For this review, take the finished solid that the model builds, in its own axes (mm). Face numbers are marked on the shaded views. A direction names the side the tool comes from. Give positions to 0.01 mm unless a question says otherwise; leave off trailing zeros. Loops run counter-clockwise (first coordinate to the right, second up) from the corner with the lowest first, then second, coordinate; pieces in that order, holes last. Notation, with made-up numbers: (60, -39.75) - (84, -39.75) arc R11 ccw to (84, -24.75) - close; hole circle Ø4 at (-25, 64). An arc over 180 degrees is marked (long way). Put each result on its own line as item: value. Start each with the question number.
Autodesk Inventor part; units mm, degrees
ref_plane "YZ Plane" through (0, 0, 0) normal (1, 0, 0) x (0, 1, 0)
ref_plane "XZ Plane" through (0, 0, 0) normal (0, 1, 0) x (-1, 0, 0)
ref_plane "XY Plane" through (0, 0, 0) normal (0, 0, 1) x (1, 0, 0)
sketch "Sketch1" plane through (0, 0, 0) normal (0, 1, 0) x (-1, 0, 0)
  line L0 (4, 2.5) -> (-4, 2.5)
  line L1 (-4, 2.5) -> (-4, -2.5)
  line L2 (-4, -2.5) -> (4, -2.5)
  line L3 (4, -2.5) -> (4, 2.5)
  line L4 (4, 2.5) -> (-4, -2.5) construction
  line L5 (-4, 2.5) -> (4, -2.5) construction
  circle A0 centre (2, 0) radius 0.889
  circle A1 centre (-1, 0) radius 0.889
  line L6 (2, -0.889) -> (-1, -0.889)
  line L7 (2, 0.889) -> (-1, 0.889)
  point P0 (0, 0)
  point P1 (0, 0)
  point P2 (0, 0)
  point P3 (0, 0)
  dimension "d19" = 8
  dimension "d20" = 5
  dimension "d21" = 1.778
  dimension "d22" = 2
  dimension "d23" = 3
extrude "Extrusion1" add sketch "Sketch1" along normal mid plane 2
sketch "Sketch4" plane through (-4, 1, 2.5) normal (0, 0, 1) x (1, 0, 0)
  line L0 (8, -2) -> (6.5, -2)
  line L1 (6.5, -2) -> (6.5, -1.5)
  line L2 (6.5, -1.5) -> (8, -1.5)
  line L3 (8, -1.5) -> (8, -2)
  line L4 (8, -2) -> (0, -2)
  line L5 (8, -2) -> (8, 0)
  point P0 (4, -1)
  dimension "d24" = 0.5
  dimension "d25" = 1.5
extrude "Extrusion3" cut sketch "Sketch4" against normal through all
fillet "Fillet2" radius 0.5 4 edges at (-4, 0, 2.5) (-4, 0, -2.5) (4, 0.25, 2.5) (4, 0.25, -2.5)
properties part number "ChipClip"
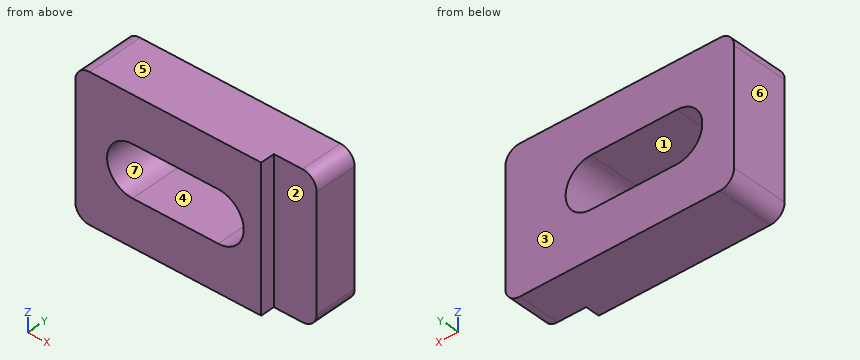
1) Mouldability with a two-part tool opening along Z and no side actions: class the marked faces 4, 5, 6 and 7 as released by +Z, released by -Z, zero draft, split by the parting line, or undercut.
2) Take a section at A-A on x = -0.5. State the section outline as (y, z) points.
3) Machinability: for the marked faces 1, 2 and 3, which of the approach directions +Z, -Z, +X, -X, +Y, -Y give a long, thin tool a straight path to every point of the face, cutting with its end or side? Answer none if there is none.
4) Take a section at C-C on z = -0.4. State the section outline as (x, y) points, and give its area (3 significant figures).
5) Wall thickness on probe 1 along Z at (x, y) = (0.75, -0.4); probe 2 along Y at (x, z) = (3, -2.2); probe 3 along X at (y, z) = (0.2, -0.5): over which ranges is each line inside the solid? List them lowest first.
6) Take a section at B-B on y = 0.9. State the section outline as (x, z) points.
7) Take a section at D-D on z = -1.8. State the section outline as (x, y) points.
8) Insertion check: P1, Ø1.6, axis at x = 3.5, z = 0.5, coming from the -Y side. The pin has a flat end and moves straight along its axis. Give the tip position at first contact, or say it passes through.
Answers follow:
1. face 4: undercut
1. face 5: released by +Z
1. face 6: zero draft
1. face 7: undercut
2. outline: (-1, -2.5) - (1, -2.5) - (1, -0.89) - (-1, -0.89) - close; (-1, 0.89) - (1, 0.89) - (1, 2.5) - (-1, 2.5) - close
3. face 1: +Y, -Y
3. face 2: +Z, -Z, +X, -Y
3. face 3: +Z, -Z, +X, -X, +Y
4. outline: (-4, -1) - (-2.79, -1) - (-2.79, 1) - (-4, 1) - close; (1.79, -1) - (2.5, -1) - (2.5, -0.5) - (4, -0.5) - (4, 1) - (1.79, 1) - close
4. area: 6.07 mm2
5. probe 1: -2.5 to -0.89, 0.89 to 2.5
5. probe 2: -0.5 to 1
5. probe 3: -4 to -2.74, 1.74 to 4
6. outline: (-4, -2) arc R0.5 ccw to (-3.5, -2.5) - (3.5, -2.5) arc R0.5 ccw to (4, -2) - (4, 2) arc R0.5 ccw to (3.5, 2.5) - (-3.5, 2.5) arc R0.5 ccw to (-4, 2) - close; hole (-2, -0.89) - (1, -0.89) arc R0.89 ccw to (1, 0.89) - (-2, 0.89) arc R0.89 ccw to start
7. outline: (-4, -1) - (2.5, -1) - (2.5, -0.5) - (4, -0.5) - (4, 1) - (-4, 1) - close
8. P1: y = -0.5
